Can you work these out from the drawing? Everything is in mm from the part's minimum corner. A direction names the side the tool comes from. Give positions to 0.01 mm unless a question says otherwise; leave off trailing zeros. Order: outer loops, then holes, each group sorted by start corner. A loop starts at its lowest first (then second) coordinate and runs counter-clockwise, first axis right, second up. Notation, with made-up numbers: M 14.25,18 L 19.25,18 A34 ccw 19.25,53 Z; hole C 34.25,35.25 d4. An arc over 180 degrees is marked long. Answer as a JSON object with one key per item and string values.
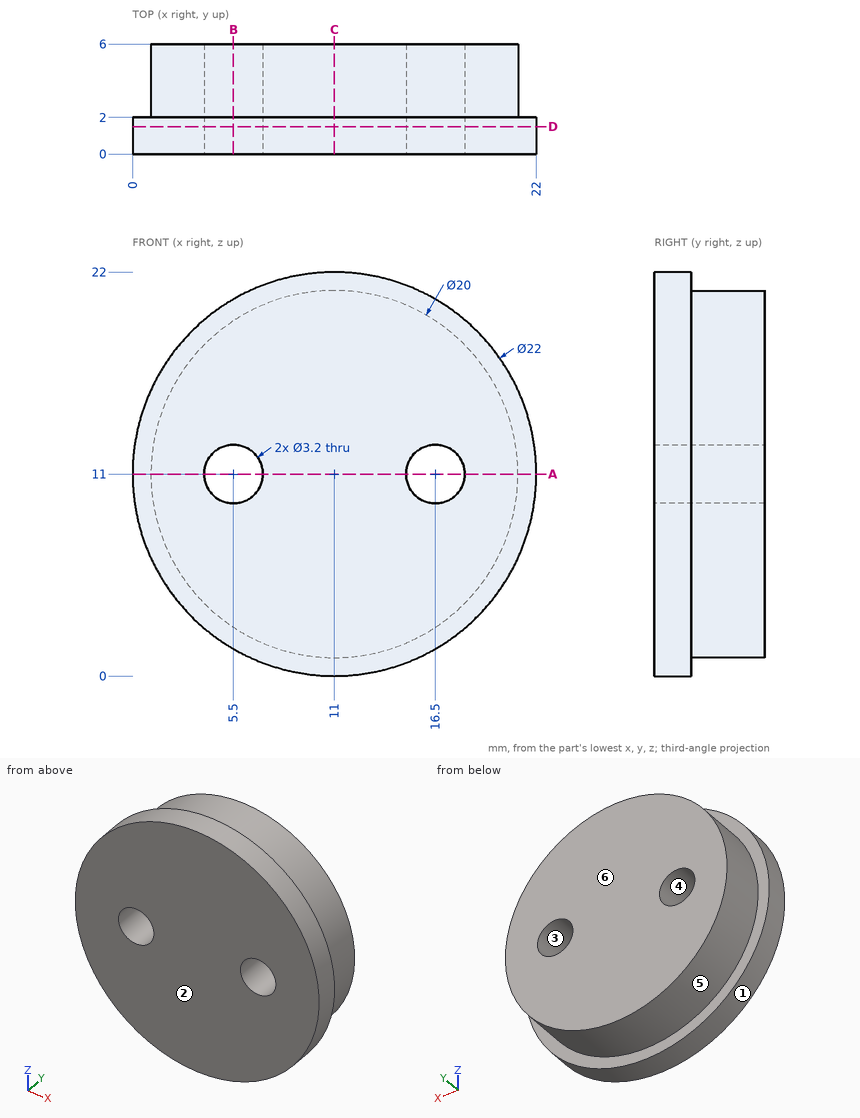
1) I want a section at A-A on z = 11. Write out the boundary of the cut face in (x, y).
Results found:
{"outline": "M 0,0 L 3.9,0 L 3.9,6 L 1,6 L 1,2 L 0,2 Z; M 7.1,0 L 14.9,0 L 14.9,6 L 7.1,6 Z; M 18.1,0 L 22,0 L 22,2 L 21,2 L 21,6 L 18.1,6 Z"}
2) I need wall thicknesses on L1, parallel to X at y = 2.05, z = 11; L2, parallel to X at y = 1.3, z = 11; L3, parallel to Z at x = 5.5, y = 1.45. Which ranges of each line are inside material? Lowest first, please.
Results found:
{"L1": "x = 1 to 3.9, 7.1 to 14.9, 18.1 to 21", "L2": "x = 0 to 3.9, 7.1 to 14.9, 18.1 to 22", "L3": "z = 1.47 to 9.4, 12.6 to 20.53"}
3) For the marked faces 5 and 6, which set-ups out of +Z, -Z, +X, -X, +Y, -Y let a thin tool reach every point of the face, with its end or its side?
Results found:
{"face 5": "+Y", "face 6": "+Z, -Z, +X, -X, +Y"}
4) I want a section at D-D on y = 1.5. Write out the boundary of the cut face in (x, z), and give its area (3 significant figures).
Results found:
{"outline": "C 11,11 d22; hole C 5.5,11 d3.2; hole C 16.5,11 d3.2", "area": "364 mm²"}
5) Thinking about a two-plate mould opening in Z: for the marked faces 1, 2, 3 and 4, which applies, pulls with the +Z half, pulls with the -Z half, needs draft (parallel to the pull), parting line crosses it, or undercut?
Results found:
{"face 1": "parting line crosses it", "face 2": "needs draft", "face 3": "undercut", "face 4": "undercut"}
6) I'm going to push flat-ended pins straight in: pin 1 Ø3 at (x, y) = (4.5, 1.5) entering from -Z; pin 2 Ø1.5 at (x, y) = (3, 1) entering from -Z. Where does each tip first touch, or does it pass through?
Results found:
{"pin 1": "stops at z = 1.2", "pin 2": "stops at z = 2.73"}
7) I want a section at B-B on x = 5.5. Write out the boundary of the cut face in (y, z), and give its area (3 significant figures).
Results found:
{"outline": "M 0,1.47 L 2,1.47 L 2,2.65 L 6,2.65 L 6,9.4 L 0,9.4 Z; M 0,12.6 L 6,12.6 L 6,19.35 L 2,19.35 L 2,20.53 L 0,20.53 Z", "area": "85.7 mm²"}
8) I want a section at C-C on x = 11. Write out the boundary of the cut face in (y, z), and give its area (3 significant figures).
Results found:
{"outline": "M 0,0 L 2,0 L 2,1 L 6,1 L 6,21 L 2,21 L 2,22 L 0,22 Z", "area": "124 mm²"}
